```python
from build123d import *

# Parameters (mm, degrees)
F0_W     = 20
F0_H     = 20
F1_DEPTH = 10
F2_T     = -1
F4_DEPTH = 9
F5_W     = 20
F5_H     = 8
F5_R     = 1.5
F6_DEPTH = 1
F7_W     = 18
F7_H     = 18
F8_DEPTH = 1
F9_R     = 0.5


with BuildPart() as f1:
    # F0 (on Top) → F1 (new body)
    with BuildSketch(Plane.XY):
        Rectangle(F0_W, F0_H)
    extrude(amount=F1_DEPTH)

    # F2
    f2_openings = [f1.faces().sort_by_distance(p)[0] for p in [
        (0, 0, 0),
    ]]
    offset(amount=F2_T, openings=f2_openings)

    # F3 (on Top) → F4 (join)
    with BuildSketch(Plane.XY):
        Polygon((-0.5, -9), (0.5, -9), (0.5, -0.5), (9, -0.5), (9, 0.5), (0.5, 0.5), (0.5, 9), (-0.5, 9), (-0.5, 0.5), (-9, 0.5), (-9, -0.5), (-0.5, -0.5), align=None)
    extrude(amount=F4_DEPTH)

    # F5 (on Top) → F6 (join)
    with BuildSketch(Plane.XY):
        with Locations((0, -13.5)):
            Rectangle(F5_W, F5_H)
        with Locations((0, -15)):
            Circle(F5_R, mode=Mode.SUBTRACT)
        with Locations((0, 14)):
            Rectangle(F5_W, F5_H)
        with Locations((0, 15)):
            Circle(F5_R, mode=Mode.SUBTRACT)
    extrude(amount=F6_DEPTH)

    # F7 (on face) → F8 (cut)
    with BuildSketch(Plane.XY.offset(10)):
        Rectangle(F7_W, F7_H)
    extrude(amount=-F8_DEPTH, mode=Mode.SUBTRACT)

    # F9
    f9_edges = [f1.edges().sort_by_distance(p)[0] for p in [
        (0, -10, 10),
        (10, 0, 10),
        (10, -10, 5.5),
        (-10, -10, 5.5),
        (-10, 0, 10),
        (0, 10, 10),
        (10, 10, 5.5),
        (-10, 10, 5.5),
    ]]
    fillet(f9_edges, radius=F9_R)


solid = f1.part
```
Read the model definition and answer for the solid it produces. Units are mm, in the model's axes. A direction names the side the tool comes from. Coordinates: 2 decimals unless noted, no trailing zeros. Order: outer loops, then holes, each group sorted by start corner. A loop starts at its lowest first (then second) coordinate and runs counter-clockwise, first axis right, second up. Notation, with made-up numbers: (-13.75, 74) - (36.25, 74) arc R10 ccw to (36.25, 86) - close; hole circle Ø11 at (56, 85.25). An arc over 180 degrees is marked (long way). Answer as a JSON object with one key per item and string values. Group by question number.
Item 1: The mould has two halves that part along Y. Classify faces 1 (the face through (10, 0, 5)), 2 (the face through (-0.1, 18, 0.5)), 3 (the face through (0.5, 5, 4)): +Y half, -Y half, draft (parallel to the pull), parting line (faces both ways), or undercut.
Item 2: Section A-A (y = 15) is taken. Give the vertices of the cut face in (x, z), plus the area to 3 significant figures.
Item 3: A tool of negligible diameter and unlimited length cuts with its end or side. For faces 4 (the face through (0, -10, 5)), 5 (the face through (5, -0.5, 4)), 6 (the face through (-10, 0, 5)), from which of +Z, -Z, +X, -X, +Y, -Y can it reach the whole face along a straight path? Write none if from no direction.
Item 4: Flat-ended cylindrical pins translate along their axes: P1, Ø4, axis at x = 5, z = 8.5, coming from the -Y side; P2, Ø4, axis at x = -4.5, y = -14, coming from the +Z side; P3, Ø4, axis at x = 1.5, z = 6.5, coming from the +Y side. Find the tip coordinate at first contact, or state that the pin passes through.
Item 5: Consider probe 1 along Y at (x, z) = (0, 0.35); probe 2 along X at (y, z) = (-5, 5.75). Determine where each line is inside the solid, lowest interval first. Write a range as from..to.
Item 6: Section D-D (y = 5.5) is taken. Give the vertices of the cut face in (x, z).
Item 7: Section B-B (x = 7.25) is taken. Give the vertices of the cut face in (y, z).
Item 8: Section C-C (z = 6) is taken. Give the vertices of the cut face in (x, y).
Results are:
{
 "1": {"face 1": "draft", "face 2": "+Y half", "face 3": "undercut"},
 "2": {"outline": "(-10, 0) - (-1.5, 0) - (-1.5, 1) - (-10, 1) - close; (1.5, 0) - (10, 0) - (10, 1) - (1.5, 1) - close", "area": "17.0 mm^2"},
 "3": {"face 4": "+Z, +X, -X, -Y", "face 5": "+Z, -Z", "face 6": "+Z, -Z, -X, +Y, -Y"},
 "4": {"P1": "stops at y = -10", "P2": "stops at z = 1", "P3": "stops at y = 10"},
 "5": {"probe 1": "y = -17.5..-16.5, -13.5..13.5, 16.5..18", "probe 2": "x = -10..-9, -0.5..0.5, 9..10"},
 "6": {"outline": "(-10, 0) - (-9, 0) - (-9, 10) - (-9.5, 10) arc R0.5 ccw to (-10, 9.5) - close; (-0.5, 0) - (0.5, 0) - (0.5, 9) - (-0.5, 9) - close; (9, 0) - (10, 0) - (10, 9.5) arc R0.5 ccw to (9.5, 10) - (9, 10) - close"},
 "7": {"outline": "(-17.5, 0) - (-9, 0) - (-9, 10) - (-9.5, 10) arc R0.5 ccw to (-10, 9.5) - (-10, 1) - (-17.5, 1) - close; (-0.5, 0) - (0.5, 0) - (0.5, 9) - (-0.5, 9) - close; (9, 0) - (18, 0) - (18, 1) - (10, 1) - (10, 9.5) arc R0.5 ccw to (9.5, 10) - (9, 10) - close"},
 "8": {"outline": "(-10, -9.5) arc R0.5 ccw to (-9.5, -10) - (9.5, -10) arc R0.5 ccw to (10, -9.5) - (10, 9.5) arc R0.5 ccw to (9.5, 10) - (-9.5, 10) arc R0.5 ccw to (-10, 9.5) - close; hole (-9, -9) - (-0.5, -9) - (-0.5, -0.5) - (-9, -0.5) - close; hole (-9, 0.5) - (-0.5, 0.5) - (-0.5, 9) - (-9, 9) - close; hole (0.5, -9) - (9, -9) - (9, -0.5) - (0.5, -0.5) - close; hole (0.5, 0.5) - (9, 0.5) - (9, 9) - (0.5, 9) - close"}
}
